Verification items for the finished model (mm, model axes). A direction names the side the tool comes from. Give positions to 0.01 mm unless a question says otherwise; leave off trailing zeros. Write each loop counter-clockwise with the first axis right and the second up, starting at its lowest first coordinate (ties: lowest second). Pieces come first, ordered by that corner, then holes. Notation, with made-up numbers: (-14.75, 2.25) - (40.25, 2.25) arc R20 cw to (40.25, 24.25) - close; hole circle Ø2 at (-24, 16.5). An arc over 180 degrees is marked (long way). Put each result on its own line as item: value.
from build123d import *

# Parameters (mm, degrees)
BOSS_EXTRUDE1_DEPTH  = 4.2
SKETCH2_W            = 6.35
SKETCH2_H            = 17.2
BOSS_EXTRUDE2_DEPTH  = 5
BOSS_EXTRUDE3_DEPTH  = 4.2
SKETCH4_W            = 0.8
SKETCH4_H            = 7.7
CUT_EXTRUDE1_DEPTH   = 0.5
SKETCH5_W            = 0.8
SKETCH5_H            = 7.7
CUT_EXTRUDE2_DEPTH   = 0.5
SKETCH6_W            = 2.7
SKETCH6_H            = 6.2
BOSS_EXTRUDE4_DEPTH  = 9.825
SKETCH7_W            = 6.7
SKETCH7_H            = 6.2
BOSS_EXTRUDE5_DEPTH  = 0.3
SKETCH8_W            = 3.13
SKETCH8_H            = 3.2
CUT_EXTRUDE3_DEPTH   = 1
SKETCH9_W            = 2.7
SKETCH9_H            = 6.2
BOSS_EXTRUDE6_DEPTH  = 9.825
SKETCH10_W           = 6.7
SKETCH10_H           = 6.2
BOSS_EXTRUDE7_DEPTH  = 0.3
SKETCH11_W           = 3.13
SKETCH11_H           = 3.2
CUT_EXTRUDE4_DEPTH   = 1
CUT_EXTRUDE5_DEPTH   = 30.55587928
CUT_EXTRUDE6_DEPTH   = 31.769302885
BOSS_EXTRUDE8_DEPTH  = 0.2
BOSS_EXTRUDE9_DEPTH  = 0.2
SKETCH16_W           = 3
SKETCH16_H           = 2.5
CUT_EXTRUDE7_DEPTH   = 0.5
SKETCH17_W           = 2.8
SKETCH17_H           = 2.3
BOSS_EXTRUDE10_DEPTH = 0.5
RIB1_START           = -0.35
RIB1_OUTLINE_W       = 0.5
RIB1_OUTLINE_H       = 7.65
RIB1_DEPTH           = 0.7
RIB2_START           = -0.35
RIB2_OUTLINE_W       = 0.5
RIB2_OUTLINE_H       = 7.65
RIB2_DEPTH           = 0.7


# Read off the part's stored shape, not the designer's step: Rib1, Rib2
with BuildPart() as part:
    # Sketch1 → Boss-Extrude1 (new body)
    with BuildSketch(Plane(origin=(-0.3, 0, 0), x_dir=(0, 0, -1), z_dir=(1, 0, 0))):
        Polygon((-12.775, 13), (-12.675, 12.9), (-12.675, -10.3), (-6.325, -10.3), (-6.325, 12.9), (-6.225, 13), (-6.325, 13.1), (-6.325, 15.9), (-12.675, 15.9), (-12.675, 13.1), align=None)
    extrude(amount=-BOSS_EXTRUDE1_DEPTH)

    # Sketch2 → Boss-Extrude2 (add)
    with BuildSketch(Plane.ZY.offset(4.5)):
        with Locations((9.5, -1.7)):
            Rectangle(SKETCH2_W, SKETCH2_H)
    extrude(amount=BOSS_EXTRUDE2_DEPTH)

    # Sketch3 → Boss-Extrude3 (add)
    with BuildSketch(Plane.ZY.offset(9.5)):
        Polygon((6.325, 13.1), (6.325, 15.9), (12.675, 15.9), (12.675, 13.1), (12.775, 13), (12.675, 12.9), (12.675, -10.3), (6.325, -10.3), (6.325, 12.9), (6.225, 13), align=None)
    extrude(amount=BOSS_EXTRUDE3_DEPTH)

    # Sketch4 → Cut-Extrude1 (cut)
    with BuildSketch(Plane(origin=(-9.5, 0, 0), x_dir=(0, 0, -1), z_dir=(1, 0, 0))):
        with Locations((-9.5, 10.75)):
            Rectangle(SKETCH4_W, SKETCH4_H)
    extrude(amount=-CUT_EXTRUDE1_DEPTH, mode=Mode.SUBTRACT)

    # Sketch5 → Cut-Extrude2 (cut)
    with BuildSketch(Plane.ZY.offset(4.5)):
        with Locations((9.5, 10.75)):
            Rectangle(SKETCH5_W, SKETCH5_H)
    extrude(amount=-CUT_EXTRUDE2_DEPTH, mode=Mode.SUBTRACT)

    # Sketch6 → Boss-Extrude4 (add)
    with BuildSketch(Plane.XY.offset(12.675)):
        with Locations((-1.65, 0)):
            Rectangle(SKETCH6_W, SKETCH6_H)
    extrude(amount=BOSS_EXTRUDE4_DEPTH)

    # Sketch7 → Boss-Extrude5 (add)
    with BuildSketch(Plane(origin=(-0.3, 0, 0), x_dir=(0, 0, -1), z_dir=(1, 0, 0))):
        with Locations((-19.15, 0)):
            Rectangle(SKETCH7_W, SKETCH7_H)
    extrude(amount=BOSS_EXTRUDE5_DEPTH)

    # Sketch8 → Cut-Extrude3 (cut)
    with BuildSketch(Plane(origin=(-0.3, 0, 0), x_dir=(0, 0, -1), z_dir=(1, 0, 0))):
        with Locations((-14.235, 0)):
            Rectangle(SKETCH8_W, SKETCH8_H)
    extrude(amount=-CUT_EXTRUDE3_DEPTH, mode=Mode.SUBTRACT)

    # Sketch9 → Boss-Extrude6 (add)
    with BuildSketch(Plane(origin=(0, 0, 6.325), x_dir=(-1, 0, 0), z_dir=(0, 0, -1))):
        with Locations((1.65, 0)):
            Rectangle(SKETCH9_W, SKETCH9_H)
    extrude(amount=BOSS_EXTRUDE6_DEPTH)

    # Sketch10 → Boss-Extrude7 (add)
    with BuildSketch(Plane(origin=(-0.3, 0, 0), x_dir=(0, 0, -1), z_dir=(1, 0, 0))):
        with Locations((0.15, 0)):
            Rectangle(SKETCH10_W, SKETCH10_H)
    extrude(amount=BOSS_EXTRUDE7_DEPTH)

    # Sketch11 → Cut-Extrude4 (cut)
    with BuildSketch(Plane(origin=(-0.3, 0, 0), x_dir=(0, 0, -1), z_dir=(1, 0, 0))):
        with Locations((-4.765, 0)):
            Rectangle(SKETCH11_W, SKETCH11_H)
    extrude(amount=-CUT_EXTRUDE4_DEPTH, mode=Mode.SUBTRACT)

    # Sketch12 → Cut-Extrude5 (cut, through all)
    with BuildSketch(Plane.ZY.offset(3)):
        with BuildLine():
            Line((18.8, -1.6), (19.9, -1.6))
            ThreePointArc((19.9, -1.6), (21.5, 0), (19.9, 1.6))
            Line((19.9, 1.6), (18.8, 1.6))
            ThreePointArc((18.8, 1.6), (17.2, 0), (18.8, -1.6))
        make_face()
    extrude(amount=-CUT_EXTRUDE5_DEPTH, mode=Mode.SUBTRACT)

    # Sketch13 → Cut-Extrude6 (cut, through all)
    with BuildSketch(Plane(origin=(0, 0, 0), x_dir=(0, 0, -1), z_dir=(1, 0, 0))):
        with BuildLine():
            Line((-0.2, -1.6), (0.9, -1.6))
            ThreePointArc((0.9, -1.6), (2.5, 0), (0.9, 1.6))
            Line((0.9, 1.6), (-0.2, 1.6))
            ThreePointArc((-0.2, 1.6), (-1.8, 0), (-0.2, -1.6))
        make_face()
    extrude(amount=-CUT_EXTRUDE6_DEPTH, mode=Mode.SUBTRACT)

    # Sketch14 → Boss-Extrude8 (add)
    with BuildSketch(Plane(origin=(0, 15.9, 0), x_dir=(-1, 0, 0), z_dir=(0, 1, 0))):
        Polygon((10.8, 10), (10.8, 9.75), (11.3, 9.75), (11.3, 9.25), (10.8, 9.25), (10.8, 9), (10.3, 9.5), align=None)
    extrude(amount=BOSS_EXTRUDE8_DEPTH)

    # Sketch15 → Boss-Extrude9 (add)
    with BuildSketch(Plane(origin=(0, 15.9, 0), x_dir=(-1, 0, 0), z_dir=(0, 1, 0))):
        Polygon((3.2, 10), (3.2, 9.75), (3.7, 9.75), (3.7, 9.25), (3.2, 9.25), (3.2, 9), (2.7, 9.5), align=None)
    extrude(amount=BOSS_EXTRUDE9_DEPTH)

    # Sketch16 → Cut-Extrude7 (cut)
    with BuildSketch(Plane.XY.offset(12.675)):
        with Locations((-8.5, -0.25)):
            Rectangle(SKETCH16_W, SKETCH16_H)
    extrude(amount=-CUT_EXTRUDE7_DEPTH, mode=Mode.SUBTRACT)

    # Sketch17 → Boss-Extrude10 (add)
    with BuildSketch(Plane.XY.offset(12.175)):
        with Locations((-8.5, -0.25)):
            Rectangle(SKETCH17_W, SKETCH17_H)
    extrude(amount=BOSS_EXTRUDE10_DEPTH)

    # Sketch18 → Revolve1 (revolve)
    with BuildSketch(Plane(origin=(0, 0, 9.5), x_dir=(-1, 0, 0), z_dir=(0, 0, -1)), mode=Mode.PRIVATE) as revolve1_sk:
        Polygon((5.6, -22.3), (7, -22.3), (7, -10.3), (4.7, -10.3), (4.7, -12.3), (5.6, -12.3), align=None)
    revolve(revolve1_sk.sketch.rotate(Axis((-7, -22.3, 9.5), (0, 1, 0)), 180), axis=Axis((-7, -22.3, 9.5), (0, 1, 0)))

    # Rib1 outline → Rib1 (add)
    with BuildSketch(Plane(origin=(0, 0, 9.5), x_dir=(-1, 0, 0), z_dir=(0, 0, -1)).offset(RIB1_START)):
        with Locations((9.75, 10.725)):
            Rectangle(RIB1_OUTLINE_W, RIB1_OUTLINE_H)
    extrude(amount=RIB1_DEPTH)

    # Rib2 outline → Rib2 (add)
    with BuildSketch(Plane.XY.offset(9.5).offset(RIB2_START)):
        with Locations((-4.25, 10.725)):
            Rectangle(RIB2_OUTLINE_W, RIB2_OUTLINE_H)
    extrude(amount=RIB2_DEPTH)


solid = part.part
Q1. Section check B-B, the plane y = 0. Give the number of separate pieces and of enclosed holes in the cut face, plus the area to 3 significant figures.
Answers follow:
separate pieces: 3
enclosed holes: 0
area: 110 mm2
Q2. Section check C-C, the plane x = -8. Record the cut outline in (y, z) (3 decimals).
Answers follow:
outline: (-22.3, 8.52) - (-12.3, 8.52) - (-12.3, 7.429) - (-10.3, 7.429) - (-10.3, 6.325) - (6.9, 6.325) - (6.9, 12.675) - (1, 12.675) - (1, 12.175) - (0.9, 12.175) - (0.9, 12.675) - (-1.4, 12.675) - (-1.4, 12.175) - (-1.5, 12.175) - (-1.5, 12.675) - (-10.3, 12.675) - (-10.3, 11.571) - (-12.3, 11.571) - (-12.3, 10.48) - (-22.3, 10.48) - close
Q3. Section check D-D, the plane y = -11. Record the cut outline in (x, z), plus the area to 3 significant figures.
Answers follow:
outline: circle Ø4.6 at (-7, 9.5)
area: 16.6 mm2
Q4. Scan lines: line 1 along Y through (x, z) = (-1, 13); line 2 along Z through (x, y) = (-10.5, -1) (3 decimals); line 3 along Y through (x, z) = (-1.25, 6.5). Record each from-to range of solid material in increasing order.
Answers follow:
line 1: y = -3.1 to -1.6, 1.6 to 3.1
line 2: z = 6.325 to 12.675
line 3: y = -10.3 to 15.9
Q5. Section check A-A, the plane y = 11. Record the cut outline in (x, z) (3 decimals), plus the area to 3 significant figures.
Answers follow:
outline: (-13.7, 6.325) - (-9.5, 6.325) - (-9.5, 9.1) - (-10, 9.1) - (-10, 9.15) - (-9.5, 9.15) - (-9.5, 9.85) - (-10, 9.85) - (-10, 9.9) - (-9.5, 9.9) - (-9.5, 12.675) - (-13.7, 12.675) - close; (-4.5, 6.325) - (-0.3, 6.325) - (-0.3, 12.675) - (-4.5, 12.675) - (-4.5, 9.9) - (-4, 9.9) - (-4, 9.85) - (-4.5, 9.85) - (-4.5, 9.15) - (-4, 9.15) - (-4, 9.1) - (-4.5, 9.1) - close
area: 53.2 mm2
Q6. Set-up check for faces 1 (the face through (-2, -3.1, 18)), 2 (the face through (-12, 14, 6.325)), 3 (the face through (-1.5, 0, -2.5)): record each of +Z, -Z, +X, -X, +Y, -Y from which the full face is reachable in a straight line by a thin tool's end or side.
Answers follow:
face 1: +Z, +X, -X, -Y
face 2: -Z, +X, -X, +Y
face 3: +X, -X
Q7. Release check for a two-part mould opening along Z. For faces 4 (the face through (-1, 1.6, 0)), 5 (the face through (-2, 14, 6.325)), 6 (the face through (-12, 15.9, 9)) record: released by +Z, released by -Z, zero draft, split by the parting line, or undercut.
Answers follow:
face 4: undercut
face 5: released by -Z
face 6: zero draft
Q8. Go/stop test with flat-tipped pins: pin 1 Ø6 at (x, y) = (-11, -16) entering from +Z; pin 2 Ø5 at (y, z) = (1.5, 16.5) entering from -X; pin 3 Ø2.5 at (x, z) = (-2, 2) entering from +Y. Record where each tip stops, or that it passes through.
Answers follow:
pin 1: stops at z = 10.48
pin 2: stops at x = -3
pin 3: stops at y = 3.1
